Can you work these out from the model? Positions are in its coordinate system, mm. Coordinates: 2 decimals unless noted, no trailing zeros. Order: outer loops, then holes, each group sorted by start corner. A loop starts at its lowest first (then second) coordinate and runs counter-clockwise, first axis right, second up. Notation, with made-up numbers: (71.25, 66.5) -> (89.25, 66.5) arc R20 cw to (89.25, 77.5) -> close; hole circle Ø5 at (-13, -6.5). An arc over 180 degrees is marked (long way). Write item = value, one per line. Start each with the question number.
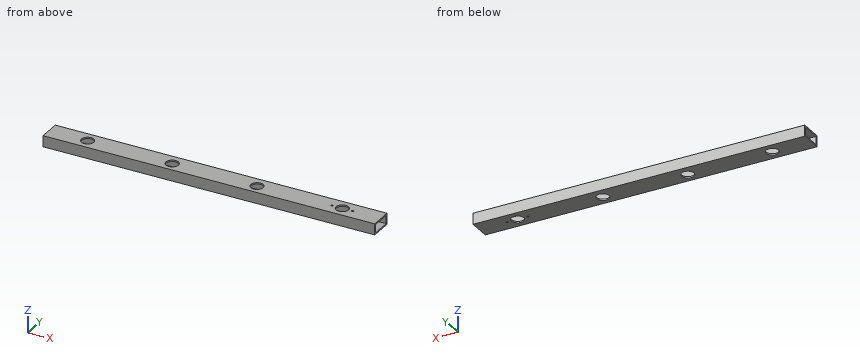
Autodesk Inventor part; units mm, degrees
ref_plane "YZ Plane" through (0, 0, 0) normal (1, 0, 0) x (0, 1, 0)
ref_plane "XZ Plane" through (0, 0, 0) normal (0, 1, 0) x (-1, 0, 0)
ref_plane "XY Plane" through (0, 0, 0) normal (0, 0, 1) x (1, 0, 0)
sketch "Sketch1" plane through (0, 0, 0) normal (0, 0, 1) x (1, 0, 0)
  line L0 (-381, -25.4) -> (381, -25.4)
  line L1 (381, -25.4) -> (381, 25.4)
  line L2 (381, 25.4) -> (-381, 25.4)
  line L3 (-381, 25.4) -> (-381, -25.4)
  line L4 (-381, -25.4) -> (381, 25.4) construction
  line L5 (381, -25.4) -> (-381, 25.4) construction
  point P0 (0, 0)
  dimension "d0" = 762
  dimension "d1" = 50.8
extrude "Extrusion1" add sketch "Sketch1" along normal blind 25.4
sketch "Sketch2" plane through (381, -25.4, 0) normal (1, 0, 0) x (0, 0, -1)
  line L0 (-25.4, 0) -> (-25.4, 50.8)
  line L1 (-25.4, 50.8) -> (0, 50.8)
  line L2 (0, 50.8) -> (0, 0)
  line L3 (0, 0) -> (-25.4, 0)
  line L4 (-25.4, 0) -> (-25.4, 50.8)
  line L5 (-3.175, 47.625) -> (-22.225, 47.625)
  line L6 (-22.225, 47.625) -> (-22.225, 3.175)
  line L7 (-22.225, 3.175) -> (-3.175, 3.175)
  line L8 (-3.175, 3.175) -> (-3.175, 47.625)
  point P0 (0, 25.4)
  dimension "d4" = 3.175
extrude "Extrusion2" cut sketch "Sketch2" against normal blind 762 contours L8 L7 L6 L5
sketch "Sketch3" plane through (0, 0, 25.4) normal (0, 0, 1) x (1, 0, 0)
  circle A0 centre (-292.5356, 0) radius 14.2875
  circle A1 centre (292.5356, 0) radius 14.2875
  line L0 (381, 25.4) -> (-381, 25.4)
  line L1 (0, 25.4) -> (0, -25.4)
  line L2 (-381, -25.4) -> (381, -25.4)
  dimension "d40" = 292.5356
  dimension "d41" = 292.5356
extrude "Extrusion3" cut sketch "Sketch3" against normal blind 25.4
sketch "Sketch5" plane through (0, 0, 25.4) normal (0, 0, 1) x (1, 0, 0)
  point P0 (0, 0)
sketch "Sketch6" plane through (0, 0, 25.4) normal (0, 0, 1) x (1, 0, 0)
  circle A0 centre (97.4989, -1.5875) radius 14.2875
  circle A1 centre (-97.4989, -1.5875) radius 14.2875
  line L0 (381, 25.4) -> (-381, 25.4)
  point P0 (0, 0)
  dimension "d28" = 97.5119
  dimension "d29" = 97.5119
  dimension "d30" = 28.575
  dimension "d31" = 28.575
  dimension "d34" = 26.9875
  dimension "d35" = 26.9875
extrude "Extrusion5" cut sketch "Sketch6" against normal blind 25.4
sketch "Sketch8" plane through (0, 0, 25.4) normal (0, 0, 1) x (1, 0, 0)
  circle A0 centre (268.7231, 0) radius 2.413
  circle A1 centre (316.3481, 0) radius 2.413
  circle A2 centre (292.5356, 0) radius 14.2875
  point P0 (0, 0)
  dimension "d42" = 47.625
  dimension "d43" = 23.8125
  dimension "d44" = 4.826
  dimension "d45" = 4.826
extrude "Extrusion7" cut sketch "Sketch8" against normal blind 25.4 contours A0 | A1
properties part number "30inchbarchassis" material "Aluminum 6061"
(1) If I drill on L1, parallel to Z at x = 319.5, y = -21 (3 decimals); L2, parallel to Y at x = 349.5, z = 4.75 (3 decimals); L3, parallel to X at y = -11, z = 22.5, over which ranges is the centre line in solid material (lowest first)? Write a range as from..to.
(2) Imagine slicing it at B-B (x = 257). Write out the boundary of the cut face in (y, z) (3 decimals), plus the area to 3 significant figures.
(3) Imagine slicing it at A-A (z = 11). Write out the boundary of the cut face in (x, y) (3 decimals), plus the area to 3 significant figures.
(4) Imagine slicing it at C-C (x = 92). Write out the boundary of the cut face in (y, z) (3 decimals), plus the area to 3 significant figures.
(5) For P1, Ø3, axis at x = 316.35, y = 0, coming from the +Z side, with a flat end and sliding along its axis, tell me the tip position at first contact or that it passes through.
Result set:
q1.L1 = 0..3.175, 22.225..25.4
q1.L2 = -25.4..-22.225, 22.225..25.4
q1.L3 = -381..-301.65, -283.42..-108.25, -86.75..86.75, 108.25..283.42, 301.65..381
q2.outline = (-25.4, 0) -> (25.4, 0) -> (25.4, 25.4) -> (-25.4, 25.4) -> close; hole (-22.225, 3.175) -> (22.225, 3.175) -> (22.225, 22.225) -> (-22.225, 22.225) -> close
q2.area = 444 mm2
q3.outline = (-381, -25.4) -> (381, -25.4) -> (381, -22.225) -> (-381, -22.225) -> close; (-381, 22.225) -> (381, 22.225) -> (381, 25.4) -> (-381, 25.4) -> close
q3.area = 4,840 mm2
q4.outline = (-25.4, 0) -> (-14.774, 0) -> (-14.774, 3.175) -> (-22.225, 3.175) -> (-22.225, 22.225) -> (-14.774, 22.225) -> (-14.774, 25.4) -> (-25.4, 25.4) -> close; (11.599, 0) -> (25.4, 0) -> (25.4, 25.4) -> (11.599, 25.4) -> (11.599, 22.225) -> (22.225, 22.225) -> (22.225, 3.175) -> (11.599, 3.175) -> close
q4.area = 276 mm2
q5.P1 = through
